Autodesk Inventor part; units mm, degrees
ref_plane "YZ Plane" through (0, 0, 0) normal (1, 0, 0) x (0, 1, 0)
ref_plane "XZ Plane" through (0, 0, 0) normal (0, 1, 0) x (-1, 0, 0)
ref_plane "XY Plane" through (0, 0, 0) normal (0, 0, 1) x (1, 0, 0)
sketch "Szkic1" plane through (0, 0, 0) normal (0, 1, 0) x (-1, 0, 0)
  line L0 (-2.4857, -2.5762) -> (1.5143, -2.5762)
  line L1 (1.5143, -2.5762) -> (1.5143, 2.4238)
  line L2 (1.5143, 2.4238) -> (-2.4857, 2.4238)
  line L3 (-3.4857, 1.4238) -> (-3.4857, -1.5762)
  arc A0 (-2.4857, 2.4238) -> (-3.4857, 1.4238) centre (-2.4857, 1.4238) ccw
  arc A1 (-3.4857, -1.5762) -> (-2.4857, -2.5762) centre (-2.4857, -1.5762) ccw
  point P0 (0, 0)
  point P1 (-3.4857, 2.4238)
  dimension "d0" = 5
  dimension "d1" = 5
  dimension "d2" = 1
extrude "Wyciągnięcie proste1" add sketch "Szkic1" along normal blind 2
sketch "Szkic2" plane through (0, 0, 0) normal (0, -1, 0) x (1, 0, 0)
  circle A0 centre (0.3828, -1.0762) radius 0.5
  circle A1 centre (0.3828, 0.9238) radius 0.5
  line L0 (2.4857, -2.5762) -> (-1.5143, -2.5762)
  line L1 (-1.5143, 2.4238) -> (2.4857, 2.4238)
  point P0 (0, 0)
  dimension "d5" = 1
  dimension "d6" = 1
  dimension "d7" = 2
  dimension "d8" = 1
  dimension "d9" = 1.5
  dimension "d10" = 1.5
extrude "Wyciągnięcie proste2" cut sketch "Szkic2" against normal blind 1
sketch "Szkic3" plane through (2.4857, 0, -2.5762) normal (0, 0, -1) x (-1, 0, 0)
  line L0 (0, 2) -> (4, 2)
  line L1 (4, 2) -> (4.2645, 3.5)
  line L2 (4.2645, 3.5) -> (2.7645, 3.5)
  line L3 (1.9737, 2) -> (4, 2)
  arc A0 (2.7645, 3.5) -> (1.9737, 2) centre (3.9714, 1.9052) ccw
  line L4 (4, 2) -> (4.7935, 6.5)
  line L5 (4.529, 5) -> (3.029, 5)
  arc A1 (3.029, 5) -> (2.7645, 3.5) centre (4.718, 3.9289) ccw
  line L6 (4.7935, 6.5) -> (3.2935, 6.5)
  arc A2 (3.2935, 6.5) -> (3.029, 5) centre (4.9825, 5.4289) ccw
  point P0 (2.4857, 0)
  point P1 (2, 2)
  point P2 (1.9737, 2)
  point P3 (3.5145, 3.5)
  dimension "d15" = 100
  dimension "d16" = 1.5
  dimension "d17" = 2
  dimension "d18" = 0
  dimension "d24" = 1.5
  dimension "d28" = 1.5
  dimension "d29" = 100
  dimension "d30" = 1.5
  dimension "d31" = 2
  dimension "d32" = 1.5
  dimension "d33" = 1.5
  dimension "d34" = 2
extrude "Wyciągnięcie proste3" add sketch "Szkic3" against normal blind 5 contours A0 L2 L1 L0
extrude "Wyciągnięcie proste4" add sketch "Szkic3" against normal blind 5 contours A1 L5 L4 L2 | A2 L6 L4 L5
fillet "Zaokrąglenie1" radius 1 1 edges at (-2.3078, 6.5, -0.0762)
properties part number "fotel" material "Tworzywo sztuczne ABS"
Geometry: final body of the model. Coordinates: model frame, mm. A direction names the side the tool comes from. Round coordinates to 2 decimals unless told otherwise and drop trailing zeros. Loops run counter-clockwise (first coordinate to the right, second up) from the corner with the lowest first, then second, coordinate; pieces in that order, holes last.
Q1. Section D-D on z = -1.3. Return loops of the section in (x, y), plus the area to 3 significant figures.
Q2. Section C-C on x = 0.75. Return loops of the section in (y, z), plus the area to 3 significant figures.
Q3. Section A-A on z = 0.2. Return loops of the section in (x, y).
Q4. Pull-direction query (Z, two-part tool) for faces 1 (the flat face through (0, 3, -2.576)), 2 (the flat face through (0.4, 1, 0.9)), 3 (the cylindrical face through (-0.265, 4.287, -0.111)), 4 (the cylindrical face through (3.201, 0.986, 2.123)); classes: released by +Z, released by -Z, zero draft, split by the parting line, or undercut.
Q5. Material intervals for L1, parallel to Y at x = 1.7, z = -1.6; L2, parallel to X at y = 1.25, z = 1.35; L3, parallel to X at y = 6.25, z = -0.7, sorted ascending.
Q6. Section B-B on y = 1.25. Return loops of the section in (x, z), plus the area to 3 significant figures.
Q7. Pin query (flat end, axial travel): P1, Ø2, axis at y = 1, z = 0, coming from the -X side; P2, Ø2, axis at y = 4.5, z = 1.5, coming from the -X side; P3, Ø1.5, axis at x = 1, z = -1.5, coming from the +Y side; P4, Ø1.5, axis at x = 2, z = 0.5, coming from the +Y side. Return the tip coordinate at first contact, or that it passes through.
Q8. Access query for faces 5 (the flat face through (0, 3, 2.424)), 6 (the flat face through (2, 2, 0)), 7 (the flat face through (-1.514, 1, 0)), 8 (the cylindrical face through (0.274, 0.493, -1.564)). Directions: +Z, -Z, +X, -X, +Y, -Y. A direction counts if a zero-diameter tool reaches every point of the face in a straight line with its end or side. Return the directions, or none.
Evaluation:
1. outline: (-2.1, 5.33) - (-1.51, 2) - (-1.51, 0) - (-0.06, 0) - (-0.06, 1) - (0.83, 1) - (0.83, 0) - (3.49, 0) - (3.49, 2) - (0.51, 2) arc R2 ccw to (-0.28, 3.5) arc R2 ccw to (-0.54, 5) arc R2 ccw to (-0.81, 6.5) - (-1.12, 6.5) arc R1 ccw to start
1. area: 16.5 mm2
2. outline: (0, -2.58) - (2, -2.58) - (2, 2.42) - (0, 2.42) - (0, 1.26) - (1, 1.26) - (1, 0.58) - (0, 0.58) - (0, -0.74) - (1, -0.74) - (1, -1.42) - (0, -1.42) - close
2. area: 8.64 mm2
3. outline: (-2.1, 5.33) - (-1.51, 2) - (-1.51, 0) - (3.49, 0) - (3.49, 2) - (0.51, 2) arc R2 ccw to (-0.28, 3.5) arc R2 ccw to (-0.54, 5) arc R2 ccw to (-0.81, 6.5) - (-1.12, 6.5) arc R1 ccw to start
4. face 1: released by -Z
4. face 2: undercut
4. face 3: zero draft
4. face 4: released by +Z
5. L1: y = 0 to 2
5. L2: x = -1.51 to 3.49
5. L3: x = -1.78 to -0.67
6. outline: (-1.51, -2.58) - (2.49, -2.58) arc R1 ccw to (3.49, -1.58) - (3.49, 1.42) arc R1 ccw to (2.49, 2.42) - (-1.51, 2.42) - close
6. area: 24.6 mm2
7. P1: stops at x = -1.51
7. P2: stops at x = -2.12
7. P3: stops at y = 2.9
7. P4: stops at y = 2
8. face 5: +Z, +X, -X, +Y, -Y
8. face 6: +Z, -Z, +X, +Y
8. face 7: +Z, -Z, -X, -Y
8. face 8: -Y
